```python
from build123d import *

# Parameters (mm, degrees)
SKETCH1_R           = 14
BOSS_EXTRUDE1_DEPTH = 20
FILLET_1_R          = 12
SKETCH2_R           = 15
BOSS_EXTRUDE2_DEPTH = 1
SKETCH3_R           = 2
BOSS_EXTRUDE3_DEPTH = 1


with BuildPart() as part:
    # Sketch1 → Boss-Extrude1 (new body)
    with BuildSketch(Plane(origin=(0, 0, 0), x_dir=(1, 0, 0), z_dir=(0, 1, 0))):
        Circle(SKETCH1_R)
    extrude(amount=BOSS_EXTRUDE1_DEPTH)

    # Fillet 1
    fillet_1_edges = [part.edges().sort_by_distance(p)[0] for p in [
        (-14, 20, 0),
    ]]
    fillet(fillet_1_edges, radius=FILLET_1_R)

    # Sketch2 → Boss-Extrude2 (add)
    with BuildSketch(Plane(origin=(0, 0, 0), x_dir=(-1, 0, 0), z_dir=(0, -1, 0))):
        Circle(SKETCH2_R)
    extrude(amount=BOSS_EXTRUDE2_DEPTH)

    # Sketch3 → Boss-Extrude3 (add)
    with BuildSketch(Plane(origin=(0, 0, 0), x_dir=(1, 0, 0), z_dir=(0, 1, 0))):
        with BuildLine():
            Line((-9.300297681, 11.768791911), (-22.328427125, 2.828427125))
            ThreePointArc((-22.328427125, 2.828427125), (-23.19551813, 1.530733729), (-23.5, 0))
            ThreePointArc((-23.5, 0), (-23.19551813, -1.530733729), (-22.328427125, -2.828427125))
            Line((-22.328427125, -2.828427125), (-9.556823766, -11.561449714))
            ThreePointArc((-9.556823766, -11.561449714), (-14.999093336, 0.164921511), (-9.300297681, 11.768791911))
        make_face()
        with Locations((-19.5, 0)):
            Circle(SKETCH3_R, mode=Mode.SUBTRACT)
        with BuildLine():
            Line((22.328427125, 2.828427125), (9.300297681, 11.768791911))
            ThreePointArc((9.300297681, 11.768791911), (13.500082689, 6.538177681), (15, 0))
            ThreePointArc((15, 0), (13.571152429, -6.389352217), (9.556823766, -11.561449714))
            Line((9.556823766, -11.561449714), (22.328427125, -2.828427125))
            ThreePointArc((22.328427125, -2.828427125), (23.19551813, -1.530733729), (23.5, 0))
            ThreePointArc((23.5, 0), (23.19551813, 1.530733729), (22.328427125, 2.828427125))
        make_face()
        with Locations((19.5, 0)):
            Circle(SKETCH3_R, mode=Mode.SUBTRACT)
    extrude(amount=-BOSS_EXTRUDE3_DEPTH)


solid = part.part
```
Geometry: final body of the model. Coordinates: model frame, mm. A direction names the side the tool comes from. Round coordinates to 2 decimals unless told otherwise and drop trailing zeros. Loops run counter-clockwise (first coordinate to the right, second up) from the corner with the lowest first, then second, coordinate; pieces in that order, holes last. Notation, with made-up numbers: (-24.5, 38) -> (-19.5, 38) arc R26 ccw to (-19.5, 68) -> close; hole circle Ø11 at (-11.75, 44). An arc over 180 degrees is marked (long way). Use one line per item in the form item = value. Start each with the question number.
1) Access query for faces 1 (the cylindrical face through (0.1, -0.5, 15)), 2 (the flat face through (-14, 0, 2.2)). Directions: +Z, -Z, +X, -X, +Y, -Y. A direction counts if a zero-diameter tool reaches every point of the face in a straight line with its end or side. Return the directions, or none.
2) Section A-A on x = -19.5. Output: boundary loops of the cut face in (y, z), then the cut area to 3 significant figures.
3) Line query: L1, parallel to X at y = 4.5, z = -0.25; L2, parallel to Z at x = -19.5, y = -0.65; L3, parallel to Y at x = -16.5, z = 0. Output: solid intervals per line, ascending.
4) First-contact query: P1, Ø5, axis at x = 9.5, z = 4, coming from the +Y side; P2, Ø4, axis at x = -8.5, z = -0.5, coming from the +Y side; P3, Ø5, axis at y = 15.5, z = -5, coming from the -X side. Flat tips, straight axial feed; report the tip coordinate or a pass-through.
Response:
q1.face_1 = +Z, +Y, -Y
q1.face_2 = +Y
q2.outline = (-1, -4.77) -> (0, -4.77) -> (0, -2) -> (-1, -2) -> close; (-1, 2) -> (0, 2) -> (0, 4.76) -> (-1, 4.76) -> close
q2.area = 5.53 mm^2
q3.L1 = -14 to 14
q3.L2 = -4.77 to -2, 2 to 4.76
q3.L3 = -1 to 0
q4.P1 = 18.5
q4.P2 = 19.12
q4.P3 = -12.18
